Verification items for the finished model (mm, model axes). A direction names the side the tool comes from. Round coordinates to 2 decimals unless told otherwise and drop trailing zeros. Order: outer loops, then holes, each group sorted by start corner. A loop starts at its lowest first (then second) coordinate and runs counter-clockwise, first axis right, second up. Notation, with made-up numbers: M 77.5,81 L 89.5,81 A25 cw 89.5,105 Z; hole C 72.25,66 d5. An arc over 180 degrees is marked long. One line per item, written item: value. Start each with the question number.
from build123d import *

# Parameters (mm, degrees)
SKETCH1_R               = 11.5
SKETCH1_R_2             = 1.05
BOSS_EXTRUDE1_DEPTH     = 4
SKETCH2_R               = 6
BOSS_EXTRUDE2_DEPTH     = 39
SKETCH3_R               = 4.25
CUT_EXTRUDE1_DEPTH      = 9
FILLET1_R               = 0.5
FILLET2_R               = 1
FILLET4_R               = 1
FILLET5_SIZE            = 7
FILLET5_SIZE_2          = 2.5
CUT_EXTRUDE2_DEPTH      = 46.972818106
CUT_EXTRUDE2_DEPTH_BACK = 46.972818106
SKETCH5_R               = 1.5


with BuildPart() as part:
    # Sketch1 → Boss-Extrude1 (new body)
    with BuildSketch(Plane.XY):
        Circle(SKETCH1_R)
        with Locations((-8, 0)):
            Circle(SKETCH1_R_2, mode=Mode.SUBTRACT)
        with Locations((0, -8)):
            Circle(SKETCH1_R_2, mode=Mode.SUBTRACT)
        with Locations((8, 0)):
            Circle(SKETCH1_R_2, mode=Mode.SUBTRACT)
        with Locations((0, 8)):
            Circle(SKETCH1_R_2, mode=Mode.SUBTRACT)
    extrude(amount=BOSS_EXTRUDE1_DEPTH)

    # Sketch2 → Boss-Extrude2 (add)
    with BuildSketch(Plane.XY.offset(4)):
        Circle(SKETCH2_R)
    extrude(amount=BOSS_EXTRUDE2_DEPTH)

    # Sketch3 → Cut-Extrude1 (cut)
    with BuildSketch(Plane(origin=(0, 0, 0), x_dir=(-1, 0, 0), z_dir=(0, 0, -1))):
        Circle(SKETCH3_R)
    extrude(amount=-CUT_EXTRUDE1_DEPTH, mode=Mode.SUBTRACT)

    # Fillet1
    fillet1_edges = [part.edges().sort_by_distance(p)[0] for p in [
        (-6, 0, 4),
        (-11.5, 0, 4),
    ]]
    fillet(fillet1_edges, radius=FILLET1_R)

    # Fillet2
    fillet2_edges = [part.edges().sort_by_distance(p)[0] for p in [
        (-6, 0, 43),
    ]]
    fillet(fillet2_edges, radius=FILLET2_R)

    # Fillet4
    fillet4_edges = [part.edges().sort_by_distance(p)[0] for p in [
        (4.25, 0, 0),
    ]]
    fillet(fillet4_edges, radius=FILLET4_R)

    # Fillet5
    # an asymmetric fillet: 7, 2.5 mm, written as the material it adds along each edge
    with BuildSketch(Plane(origin=(0, 0, 9), x_dir=(-1, 0, 0), z_dir=(0, -1, 0))) as fillet5_piece_1:
        with BuildLine():
            Bezier((4.25, FILLET5_SIZE), (4.25, 0), (4.25 - FILLET5_SIZE_2, 0), weights=[1, 0.707106781, 1])
            Line((4.25 - FILLET5_SIZE_2, 0), (4.25, 0))
            Line((4.25, 0), (4.25, FILLET5_SIZE))
        make_face()
    revolve(axis=Axis((0, 0, 9), (0, 0, -1)))

    # Sketch5 → Cut-Extrude2 (cut, two sides: drawn at the far end of the back side and taken through both)
    with BuildSketch(Plane(origin=(0, 0, 0), x_dir=(1, 0, 0), z_dir=(0, 1, 0)).offset(-CUT_EXTRUDE2_DEPTH_BACK)):
        with Locations(Location((0, -36.5, 0), (0, 0, 270))):
            Circle(SKETCH5_R)
    extrude(amount=CUT_EXTRUDE2_DEPTH + CUT_EXTRUDE2_DEPTH_BACK, mode=Mode.SUBTRACT)


solid = part.part
1. Scan lines: line 1 along Z through (x, y) = (-1.5, -9); line 2 along Y through (x, z) = (0, 3.2); line 3 along X through (y, z) = (2.5, 36.5). Record each from-to range of solid material in increasing order.
2. Section check D-D (z = 36.5). Record the cut outline in (x, y), and give its area (3 significant figures).
3. Depth check by flat-ended pin: pin 1 (4 mm diameter, centred on x = -0.5, y = 0.5, fed in from -Z); pin 2 (1 mm diameter, centred on x = -8.5, y = 5.5, fed in from -Z); pin 3 (8 mm diameter, centred on y = -5.5, z = 18, fed in from +X); pin 4 (5 mm diameter, centred on x = 3.5, z = 31.5, fed in from +Y). Enter the tip coordinate at first touch or a pass-through.
4. Tool access check on faces 1 (the face through (-1.301, -5.857, 22.988)), 2 (the face through (-2.285, 3.584, 1.493)), 3 (the face through (0, 0, 43)). Record the directions out of +Z, -Z, +X, -X, +Y, -Y that give a thin tool (end or side, any length) a straight path to the whole face; none if there is none.
5. Draft check along Y on faces 4 (the face through (-1.5, 11.4, 1.7)), 5 (the face through (5, -5, 4)), 6 (the face through (0, 0, 9)). Enter one of: released by +Y, released by -Y, zero draft, split by the parting line, or undercut.
6. Section check A-A (y = 0). Give the number of separate pieces and of enclosed holes in the cut face, and give its area (3 significant figures).
7. Section check C-C (z = 25.5). Record the cut outline in (x, y), and give its area (3 significant figures).
Geometry check:
1. line 1: z = 0 to 4
1. line 2: y = -11.5 to -9.05, -6.95 to -4.21, 4.21 to 6.95, 9.05 to 11.5
1. line 3: x = -5.45 to -1.5, 1.5 to 5.45
2. outline: M -1.5,-5.81 L -1.5,5.81 A6 ccw Z; M 1.5,-5.81 A6 ccw 1.5,5.81 Z
2. area: 77.5 mm²
3. pin 1: stops at z = 8.47
3. pin 2: stops at z = 0
3. pin 3: stops at x = 5.81
3. pin 4: stops at y = 5.92
4. face 1: +Z
4. face 2: -Z
4. face 3: +Z, +X, -X, +Y, -Y
5. face 4: split by the parting line
5. face 5: zero draft
5. face 6: undercut
6. separate pieces: 3
6. enclosed holes: 1
6. area: 466 mm²
7. outline: C 0,0 d12
7. area: 113 mm²
